```python
from build123d import *

# Parameters (mm, degrees)
SKETCH1_W            = 25
SKETCH1_H            = 20.5
BOSS_EXTRUDE1_DEPTH  = 1.2
USB_START            = 1.9
SKETCH2_W            = 3.6
SKETCH2_H            = 7
USB_CONNECTOR_DEPTH  = 10
SKETCH3_W            = 1.8
SKETCH3_H            = 3.3
MICROPROCESSOR_DEPTH = 1.8
SKETCH4_W            = 5
SKETCH4_H            = 4
BUTTON_BASE_DEPTH    = 1.1


with BuildPart() as part:
    # Sketch1 → Boss-Extrude1 (new body)
    with BuildSketch(Plane.XY):
        Rectangle(SKETCH1_W, SKETCH1_H)
    extrude(amount=BOSS_EXTRUDE1_DEPTH)

    # Sketch2 → USB Connector (add)
    with BuildSketch(Plane.ZY.offset(12.5).offset(USB_START)):
        with Locations((3, 0)):
            Rectangle(SKETCH2_W, SKETCH2_H)
    extrude(amount=-USB_CONNECTOR_DEPTH)

    # Sketch3 → MicroProcessor (add)
    with BuildSketch(Plane.XY.offset(1.2)):
        with Locations((11.6, -0.9)):
            Rectangle(SKETCH3_W, SKETCH3_H)
    extrude(amount=MICROPROCESSOR_DEPTH)

    # Sketch4 → Button Base (add)
    with BuildSketch(Plane.XY.offset(1.2)):
        with Locations((4, -5.25)):
            Rectangle(SKETCH4_W, SKETCH4_H)
    extrude(amount=BUTTON_BASE_DEPTH)


solid = part.part
```
Can you work these out from the model? Positions are in its coordinate system, mm. A direction names the side the tool comes from. Coordinates: 2 decimals unless noted, no trailing zeros. Loops run counter-clockwise (first coordinate to the right, second up) from the corner with the lowest first, then second, coordinate; pieces in that order, holes last. Notation, with made-up numbers: M 53,-26 L 68,-26 A19 cw 68,-21 Z; hole C -22.5,-27 d8. An arc over 180 degrees is marked long. Put each result on its own line as item: value. Start each with the question number.
(1) Which directions (+Z, -Z, +X, -X, +Y, -Y) give clear straight access to the entire face, cutting with the end or side of a thin tool? Please do faces 5 (the face through (-13, 0, 1.2)), 6 (the face through (12, -2.55, 2)), 7 (the face through (4, -3.25, 2)), 8 (the face through (4, -7.25, 2)), 9 (the face through (-9, -3.5, 3)).
(2) Imagine slicing it at A-A on y = 1.75. List the corners of the cut face in (x, z) for me, and give its area (3 significant figures).
(3) Imagine slicing it at C-C on z = 0.8. List the corners of the cut face in (x, y) for me, and give its area (4 significant figures).
(4) Imagine slicing it at D-D on y = -1.5. List the corners of the cut face in (x, z) for me, and give its area (3 significant figures).
(5) Will these pins go through, and if not, where does the flat tip stop? pin 1 Ø3 at (x, y) = (5, -5.5) entering from +Z; pin 2 Ø5 at (x, y) = (8, 0) entering from +Z; pin 3 Ø1.4 at (x, z) = (11.5, 2) entering from +Y.
(6) I need wall thicknesses on probe 1 along X at (y, z) = (0, 1.5); probe 2 along Z at (x, y) = (2.75, -2.5); probe 3 along Y at (x, z) = (5.75, 1.45). Which ranges of each line are inside material? Lowest first, please.
(7) We'd pull the mould along X, two halves only. Please class faces 1 (the face through (10.7, -1, 2)), 2 (the face through (12, 0.75, 2)), 3 (the face through (6.5, -5, 2)), 4 (the face through (-12.5, 0, 1)): +X half, -X half, draft (parallel to the pull), parting line (faces both ways), or undercut.
(8) Imagine slicing it at B-B on x = -5. List the corners of the cut face in (y, z) for me.
Worked answers:
1. face 5: -Z, -X, +Y, -Y
1. face 6: +Z, +X, -Y
1. face 7: +Z, +X, +Y
1. face 8: +Z, +X, -X, -Y
1. face 9: +Z, -X, -Y
2. outline: M -14.4,1.2 L -12.5,1.2 L -12.5,0 L 12.5,0 L 12.5,1.2 L -4.4,1.2 L -4.4,4.8 L -14.4,4.8 Z
2. area: 66.0 mm2
3. outline: M -12.5,-10.25 L 12.5,-10.25 L 12.5,10.25 L -12.5,10.25 Z
3. area: 512.5 mm2
4. outline: M -14.4,1.2 L -12.5,1.2 L -12.5,0 L 12.5,0 L 12.5,3 L 10.7,3 L 10.7,1.2 L -4.4,1.2 L -4.4,4.8 L -14.4,4.8 Z
4. area: 69.2 mm2
5. pin 1: stops at z = 2.3
5. pin 2: stops at z = 1.2
5. pin 3: stops at y = 0.75
6. probe 1: x = -14.4 to -4.4, 10.7 to 12.5
6. probe 2: z = 0 to 1.2
6. probe 3: y = -7.25 to -3.25
7. face 1: undercut
7. face 2: draft
7. face 3: +X half
7. face 4: -X half
8. outline: M -10.25,0 L 10.25,0 L 10.25,1.2 L 3.5,1.2 L 3.5,4.8 L -3.5,4.8 L -3.5,1.2 L -10.25,1.2 Z
